Build history of the part. All positions in model axes, mm. A direction names the side the tool comes from. Round coordinates to 2 decimals unless told otherwise and drop trailing zeros. Order: outer loops, then holes, each group sorted by start corner. A loop starts at its lowest first (then second) coordinate and runs counter-clockwise, first axis right, second up. Notation, with made-up numbers: (14, 53) - (57, 53) arc R38 ccw to (57, 92) - close; hole circle Ø1 at (-38.75, 33.5). An arc over 180 degrees is marked (long way). One line per question, with ' | ' between items. Start each with the question number.
from build123d import *

# Parameters (mm, degrees)
F0_W      = 60
F0_H      = 50
F0_R      = 22
F0_R_2    = 18.5
F0_R_3    = 13.5
F0_H_2    = 5
F1_DEPTH  = 8.89
F2_DEPTH  = 35
F3_W      = 30
F3_H      = 5
F4_DEPTH  = 60
F5_R      = 5
F6_R      = 9.025
F7_DEPTH  = 7.112
F8_DEPTH  = 25
F6_R_2    = 9.525
F9_DEPTH  = 7.112
F10_R     = 10
F12_DEPTH = 30
F13_R     = 18.5
F14_DEPTH = 22
F15_R     = 2.5275
F16_DEPTH = 13
F17_R     = 3.175
F18_DEPTH = 25


with BuildPart() as f1:
    # F0 (on Front) → F1 (new body)
    with BuildSketch(Plane.XZ):
        Rectangle(F0_W, F0_H)
        Circle(F0_R, mode=Mode.SUBTRACT)
        Circle(F0_R)
        Circle(F0_R_2, mode=Mode.SUBTRACT)
        Circle(F0_R_2)
        Circle(F0_R_3, mode=Mode.SUBTRACT)
        with Locations((0, -27.5)):
            Rectangle(F0_W, F0_H_2)
    extrude(amount=F1_DEPTH)

    # F0 (on Front) → F2 (join)
    with BuildSketch(Plane.XZ):
        Circle(F0_R)
        Circle(F0_R_2, mode=Mode.SUBTRACT)
    extrude(amount=F2_DEPTH)

    # F3 (on face) → F4 (join)
    with BuildSketch(Plane.YZ.offset(30)):
        Polygon((30, -25), (30, -30), (38.89, -30), (38.89, 25), (30, 25), align=None)
        with Locations((15, -27.5)):
            Rectangle(F3_W, F3_H)
    extrude(amount=-F4_DEPTH)

    # F5
    f5_edges = [f1.edges().sort_by_distance(p)[0] for p in [
        (0, 30, -25),
        (0, 0, -25),
    ]]
    fillet(f5_edges, radius=F5_R)

    # F6 (on face) → F7 (cut)
    with BuildSketch(Plane(origin=(0, 38.89, 0), x_dir=(-1, 0, 0), z_dir=(0, 1, 0))):
        Circle(F6_R)
    extrude(amount=-F7_DEPTH, mode=Mode.SUBTRACT)

    # F6 (on face) → F8 (cut)
    with BuildSketch(Plane(origin=(0, 38.89, 0), x_dir=(-1, 0, 0), z_dir=(0, 1, 0))):
        Circle(F6_R)
    extrude(amount=-F8_DEPTH, mode=Mode.SUBTRACT)

    # F6 (on face) → F9 (cut)
    with BuildSketch(Plane(origin=(0, 38.89, 0), x_dir=(-1, 0, 0), z_dir=(0, 1, 0))):
        Circle(F6_R_2)
        Circle(F6_R, mode=Mode.SUBTRACT)
    extrude(amount=-F9_DEPTH, mode=Mode.SUBTRACT)

    # F10
    f10_edges = [f1.edges().sort_by_distance(p)[0] for p in [
        (30, -4.445, 25),
        (30, 34.445, 25),
        (-30, -4.445, 25),
        (-30, 34.445, 25),
    ]]
    fillet(f10_edges, radius=F10_R)

    # F11 (on Right) → F12 (join)
    with BuildSketch(Plane.YZ):
        with BuildLine():
            ThreePointArc((-21.5492570434, 7.385385089), (-29.0335155473, 0.0988734149), (-21.7470038732, -7.385385089))
            Line((-21.7470038732, -7.385385089), (-21.5492570434, 7.385385089))
        make_face()
        with BuildLine():
            Line((-21.5492570434, 7.385385089), (-21.7470038732, -7.385385089))
            ThreePointArc((-21.7470038732, -7.385385089), (-16.4604814154, -5.2575646712), (-14.2620835546, 0))
            ThreePointArc((-14.2620835546, 0), (-16.3905657871, 5.1876490429), (-21.5492570434, 7.385385089))
        make_face()
    extrude(amount=-F12_DEPTH)

    # F13 (on face) → F14 (cut)
    with BuildSketch(Plane.XZ.offset(35)):
        Circle(F13_R)
    extrude(amount=-F14_DEPTH, mode=Mode.SUBTRACT)

    # F15 (on face) → F16 (cut)
    with BuildSketch(Plane(origin=(-30, 0, 0), x_dir=(0, -1, 0), z_dir=(-1, 0, 0))):
        with Locations((21.6481304583, 0)):
            Circle(F15_R)
    extrude(amount=-F16_DEPTH, mode=Mode.SUBTRACT)

    # F17 (on face) → F18 (cut)
    with BuildSketch(Plane(origin=(0, 0, -30), x_dir=(1, 0, 0), z_dir=(0, 0, -1))):
        with Locations((-15, -15)):
            Circle(F17_R)
        with Locations((15, -15)):
            Circle(F17_R)
    extrude(amount=-F18_DEPTH, mode=Mode.SUBTRACT)


solid = f1.part
Item 1: Wall check: line 1 along Y through (x, z) = (-15, -27) (3 decimals); line 2 along X through (y, z) = (15, -28.4) (3 decimals); line 3 along Z through (x, y) = (0, 37) (3 decimals). Give the ranges that are in metal, low to high. Write a range as [from, to].
Item 2: Pull direction X, two halves, no side cores. Call faces 1 (the face through (-30, 31, -7)), 2 (the face through (0, -4, 25)), 3 (the face through (-11.97, 14.05, -27.54)), 4 (the face through (18.03, 14.05, -27.54)): released by +X, released by -X, zero draft, split by the parting line, or undercut.
Item 3: Slice it at A-A (x = 0). Count the separate pieces of the cut face and the enclosed holes in it, plus the area to 3 significant figures.
Item 4: Pin check, flat tips, straight feed: pin 1 (5.5 mm diameter, centred on x = 15, y = 15, fed in from -Z); pin 2 (4 mm diameter, centred on y = -22.5, z = 1, fed in from +X); pin 3 (21 mm diameter, centred on x = 0, z = 0, fed in from -Y); pin 4 (22 mm diameter, centred on x = 12, y = 18, fed in from +Z). Stop position of each tip, or through.
Item 5: Slice it at C-C (y = -8). Write the cut outline in (x, z).
Item 6: Slice it at D-D (x = 15). Write the cut outline in (y, z) (3 decimals).
Item 7: Slice it at B-B (z = -16). Write the cut outline in (x, y).
Item 8: 3-axis set-ups, long thin cutter, end or side, ignore diameter. For faces 5 (the face through (-7, 0, 13)), 6 (the face through (-2.93, -4.38, -13.18)), 7 (the face through (-7, 31.778, 6)): which of +Z, -Z, +X, -X, +Y, -Y reach the whole face in a straight line?
A:
1) line 1: [-8.89, 11.825], [18.175, 38.89] | line 2: [-30, -18.175], [-11.825, 11.825], [18.175, 30] | line 3: [-30, -9.525], [9.525, 25]
2) face 1: released by -X | face 2: zero draft | face 3: undercut | face 4: undercut
3) separate pieces: 3 | enclosed holes: 0 | area: 914 mm^2
4) pin 1: through | pin 2: x = 22 | pin 3: y = 30 | pin 4: z = -23
5) outline: (-30, -30) - (30, -30) - (30, 15) arc R10 ccw to (20, 25) - (-20, 25) arc R10 ccw to (-30, 15) - close; hole circle Ø27 at (0, 0)
6) outline: (-35, -16.093) - (-8.89, -16.093) - (-8.89, -30) - (11.825, -30) - (11.825, -25) - (5, -25) arc R5 cw to (0, -20) - (0, 25) - (-8.89, 25) - (-8.89, 16.093) - (-35, 16.093) - (-35, 10.828) - (-8.89, 10.828) - (-8.89, -10.828) - (-35, -10.828) - close; (18.175, -30) - (38.89, -30) - (38.89, 25) - (30, 25) - (30, -20) arc R5 cw to (25, -25) - (18.175, -25) - close
7) outline: (-30, -8.89) - (-15.1, -8.89) - (-15.1, -35) - (-9.29, -35) - (-9.29, -8.89) - (9.29, -8.89) - (9.29, -35) - (15.1, -35) - (15.1, -8.89) - (30, -8.89) - (30, 0) - (-30, 0) - close; (-30, 30) - (30, 30) - (30, 38.89) - (-30, 38.89) - close
8) face 5: +Z, +X, -X | face 6: -Y | face 7: +Y
